from build123d import *

# Parameters (mm, degrees)
AUFSATZ_LINEAR_AUSTRAGEN1_DEPTH      = 10
SKIZZE6_R                            = 1.9
SKIZZE6_R_2                          = 11.25
SCHNITT_LINEAR_AUSTRAGEN4_DEPTH      = 67.632124385
SKIZZE7_W                            = 20.880821379
SKIZZE7_H                            = 5
SCHNITT_LINEAR_AUSTRAGEN5_DEPTH      = 87.970339772
VERRUNDUNG3_R                        = 15
SCHNITT_LINEAR_AUSTRAGEN6_DEPTH      = 69.731361244
SCHNITT_LINEAR_AUSTRAGEN6_DEPTH_BACK = 69.731361244
SKIZZE8_W                            = 10
SKIZZE8_H                            = 5
SKIZZE9_R                            = 1.7
SCHNITT_LINEAR_AUSTRAGEN7_DEPTH      = 10
AUFSATZ_LINEAR_AUSTRAGEN2_DEPTH      = 5


with BuildPart() as part:
    # Skizze1 → Aufsatz-Linear austragen1 (new body)
    with BuildSketch(Plane(origin=(0, 0, 0), x_dir=(1, 0, 0), z_dir=(0, 1, 0))):
        Polygon((-60, -4.8), (-22, -4.8), (-22, -16.8), (22, -16.8), (22, -4.8), (60, -4.8), (60, 15.2), (22, 15.2), (22, 27.2), (0, 27.2), (-22, 27.2), (-22, 15.2), (-60, 15.2), align=None)
    extrude(amount=AUFSATZ_LINEAR_AUSTRAGEN1_DEPTH)

    # Skizze6 → Schnitt-Linear austragen4 (cut, through all)
    with BuildSketch(Plane(origin=(0, 10, 0), x_dir=(1, 0, 0), z_dir=(0, 1, 0))):
        with Locations(Location((15.5, 20.7, 0), (0, 0, 270))):
            Circle(SKIZZE6_R)
        with Locations(Location((15.5, -10.3, 0), (0, 0, 270))):
            Circle(SKIZZE6_R)
        with Locations(Location((-15.5, -10.3, 0), (0, 0, 270))):
            Circle(SKIZZE6_R)
        with Locations(Location((-15.5, 20.7, 0), (0, 0, 270))):
            Circle(SKIZZE6_R)
        with Locations(Location((0, 5.2, 0), (0, 0, 270))):
            Circle(SKIZZE6_R_2)
    extrude(amount=-SCHNITT_LINEAR_AUSTRAGEN4_DEPTH, mode=Mode.SUBTRACT)

    # Skizze7 → Schnitt-Linear austragen5 (cut, through all)
    with BuildSketch(Plane.ZY.offset(22)):
        with Locations((-25.64041069, 2.5)):
            Rectangle(SKIZZE7_W, SKIZZE7_H)
    extrude(amount=-SCHNITT_LINEAR_AUSTRAGEN5_DEPTH, mode=Mode.SUBTRACT)

    # Verrundung3
    # the kernel refuses this fillet: 15 mm, written as the material it adds along each edge
    with BuildSketch(Plane(origin=(-22, 5, -15.2), x_dir=(0, 0, -1), z_dir=(0, 1, 0))) as verrundung3_piece_1:
        with BuildLine():
            CenterArc((15, 14.696938457), VERRUNDUNG3_R, 180, 78.463040967)
            Line((0, 14.696938457), (-0.3, 14.696938457))
            Line((-0.3, 14.696938457), (-0.3, 0))
            Line((-0.3, 0), (0, -0.3))
            ThreePointArc((0, -0.3), (6, -0.3), (11.94, -0.293938769))
            Line((11.94, -0.293938769), (12, 0))
        make_face()
    extrude(amount=5)
    with BuildSketch(Plane(origin=(-22, 0, 4.8), x_dir=(-1, 0, 0), z_dir=(0, 1, 0))) as verrundung3_piece_2:
        with BuildLine():
            CenterArc((14.696938457, 15), VERRUNDUNG3_R, 191.536959033, 78.463040967)
            Line((0, 12), (-0.293938769, 11.94))
            ThreePointArc((-0.293938769, 11.94), (-0.3, 6), (-0.3, 0))
            Line((-0.3, 0), (0, -0.3))
            Line((0, -0.3), (14.696938457, -0.3))
            Line((14.696938457, -0.3), (14.696938457, 0))
        make_face()
    extrude(amount=10)
    with BuildSketch(Plane(origin=(22, 0, 4.8), x_dir=(1, 0, 0), z_dir=(0, 1, 0))) as verrundung3_piece_3:
        with BuildLine():
            CenterArc((14.696938457, -15), VERRUNDUNG3_R, 90, 78.463040967)
            Line((0, -12), (-0.293938769, -11.94))
            ThreePointArc((-0.293938769, -11.94), (-0.3, -6), (-0.3, 0))
            Line((-0.3, 0), (0, 0.3))
            Line((0, 0.3), (14.696938457, 0.3))
            Line((14.696938457, 0.3), (14.696938457, 0))
        make_face()
    extrude(amount=10)
    with BuildSketch(Plane(origin=(22, 5, -15.2), x_dir=(1, 0, 0), z_dir=(0, 1, 0))) as verrundung3_piece_4:
        with BuildLine():
            CenterArc((14.696938457, 15), VERRUNDUNG3_R, 191.536959033, 78.463040967)
            Line((0, 12), (-0.293938769, 11.94))
            ThreePointArc((-0.293938769, 11.94), (-0.3, 6), (-0.3, 0))
            Line((-0.3, 0), (0, -0.3))
            Line((0, -0.3), (14.696938457, -0.3))
            Line((14.696938457, -0.3), (14.696938457, 0))
        make_face()
    extrude(amount=5)

    # Verrundung4
    # a fillet whose section is not a circle: 17 mm, written as the material it takes off along each edge
    with BuildSketch(Plane(origin=(-5.153882032, -55.537810403, -15.2), x_dir=(-0.4098221227148323, 0, 0.912165460721633), z_dir=(0, 1, 0))) as verrundung4_piece_1:
        with BuildLine():
            Bezier((14.018959465, 0), (3.694910003, -8.223980839), (9.10424934, -20.263868965), weights=[1, 0.223796354, 1])
            Line((9.10424934, -20.263868965), (0, 0))
            ThreePointArc((0, 0), (7.009479733, -2.450585595), (14.018959465, 0))
        make_face()
    extrude(amount=60.537810403, mode=Mode.SUBTRACT)
    with BuildSketch(Plane(origin=(5.153882032, -55.537810403, -15.2), x_dir=(0.40982212271483137, 0, 0.9121654607216333), z_dir=(0, 1, 0))) as verrundung4_piece_2:
        with BuildLine():
            Bezier((14.018959465, 0), (3.694910003, 8.223980839), (9.10424934, 20.263868965), weights=[1, 0.223796354, 1])
            Line((9.10424934, 20.263868965), (0, 0))
            ThreePointArc((0, 0), (7.009479733, 2.450585595), (14.018959465, 0))
        make_face()
    extrude(amount=60.537810403, mode=Mode.SUBTRACT)

    # Skizze8 → Schnitt-Linear austragen6 (cut, two sides: drawn at the far end of the back side and taken through both)
    with BuildSketch(Plane(origin=(0, 0, -15.2), x_dir=(-1, 0, 0), z_dir=(0, 0, -1)).offset(-SCHNITT_LINEAR_AUSTRAGEN6_DEPTH_BACK)):
        with Locations((-55, 2.5)):
            Rectangle(SKIZZE8_W, SKIZZE8_H)
        with Locations((55, 2.5)):
            Rectangle(SKIZZE8_W, SKIZZE8_H)
    extrude(amount=SCHNITT_LINEAR_AUSTRAGEN6_DEPTH + SCHNITT_LINEAR_AUSTRAGEN6_DEPTH_BACK, mode=Mode.SUBTRACT)

    # Skizze9 → Schnitt-Linear austragen7 (cut)
    with BuildSketch(Plane.XZ.offset(-5)):
        with Locations(Location((-55, -0.2, 0), (0, 0, 270))):
            Circle(SKIZZE9_R)
        with Locations(Location((-55, -10.2, 0), (0, 0, 90))):
            Circle(SKIZZE9_R)
        with Locations(Location((55, -10.2, 0), (0, 0, 270))):
            Circle(SKIZZE9_R)
        with Locations(Location((55, -0.2, 0), (0, 0, 90))):
            Circle(SKIZZE9_R)
    extrude(amount=-SCHNITT_LINEAR_AUSTRAGEN7_DEPTH, mode=Mode.SUBTRACT)

    # Skizze10 → Aufsatz-Linear austragen2 (add)
    with BuildSketch(Plane(origin=(0, 10, 0), x_dir=(1, 0, 0), z_dir=(0, 1, 0))):
        Polygon((-22, 27.2), (-20.360366379, 30.307150274), (-18.720732758, 27.2), align=None)
    extrude(amount=-AUFSATZ_LINEAR_AUSTRAGEN2_DEPTH)


solid = part.part
Verification items for the finished model (mm, model axes). A direction names the side the tool comes from. Give positions to 0.01 mm unless a question says otherwise; leave off trailing zeros. Write each loop counter-clockwise with the first axis right and the second up, starting at its lowest first coordinate (ties: lowest second). Pieces come first, ordered by that corner, then holes.
(1) Cross-section at D-D (z = -0.2). Enter the section's corners in (x, y), plus the area to 3 significant figures.
(2) Cross-section at B-B (z = 10.3). Enter the section's corners in (x, y).
(3) Gauge pin test, flat ends, axial feed: pin 1 (5.5 mm diameter, centred on x = 5, y = 6.5, fed in from -Z); pin 2 (5 mm diameter, centred on x = 37, y = 7, fed in from -Z); pin 3 (5.5 mm diameter, centred on x = 55, z = -0.2, fed in from -Y). Record the tip position at first contact, or that the pin passes through.
(4) Cross-section at A-A (y = 7). State how many separate pieces and enclosed holes the cut face has, plus the area to 3 significant figures.
(5) Material ranges on line 1 (X direction, y = 6, z = -0.2); line 2 (X direction, y = 8.25, z = -20.5); line 3 (Y direction, x = -53, z = -7), recorded low to high.
(6) Cross-section at C-C (x = -55). Enter the section's corners in (y, z), plus the area to 3 significant figures.
(7) Mould release check, pull along Z, two halves, no side actions. Record for faces 5 (the face through (-56.15, 7.46, -11.45)), 6 (the face through (55.07, 7.46, -8.5)), 7 (the face through (0, 5, 16.8)), 8 (the face through (1, 0, 8)): +Z half, -Z half, draft (parallel to the pull), parting line (faces both ways), or undercut.
(8) Access from +Z, -Z, +X, -X, +Y, -Y to the whole of each face (thin tool, end or side, straight path). Record for faces 1 (the face through (0, 5, -18)), 2 (the face through (43, 5, -15.2)), 3 (the face through (-46, 6, 4.8)), 4 (the face through (46, 6, 4.8)).
Worked out:
1. outline: (-60, 5) - (-56.7, 5) - (-56.7, 10) - (-60, 10) - close; (-53.3, 5) - (-50, 5) - (-50, 0) - (-10.08, 0) - (-10.08, 10) - (-53.3, 10) - close; (10.08, 0) - (50, 0) - (50, 5) - (53.3, 5) - (53.3, 10) - (10.08, 10) - close; (56.7, 5) - (60, 5) - (60, 10) - (56.7, 10) - close
1. area: 864 mm2
2. outline: (-25.09, 0) - (-17.4, 0) - (-17.4, 10) - (-25.09, 10) - close; (-13.6, 0) - (13.6, 0) - (13.6, 10) - (-13.6, 10) - close; (17.4, 0) - (25.09, 0) - (25.09, 10) - (17.4, 10) - close
3. pin 1: stops at z = -27.2
3. pin 2: stops at z = -15.36
3. pin 3: stops at y = 5
4. separate pieces: 1
4. enclosed holes: 9
4. area: 3,160 mm2
5. line 1: x = -60 to -56.7, -53.3 to -10.08, 10.08 to 53.3, 56.7 to 60
5. line 2: x = -25.26 to -17.39, -13.61 to 13.61, 17.39 to 25.26
5. line 3: y = 5 to 10
6. outline: (5, -15.2) - (10, -15.2) - (10, -11.9) - (5, -11.9) - close; (5, -8.5) - (10, -8.5) - (10, -1.9) - (5, -1.9) - close; (5, 1.5) - (10, 1.5) - (10, 4.8) - (5, 4.8) - close
6. area: 66.0 mm2
7. face 5: undercut
7. face 6: undercut
7. face 7: +Z half
7. face 8: draft
8. face 1: -Z, -Y
8. face 2: -Z, +X, -Y
8. face 3: +Z, -X, +Y, -Y
8. face 4: +Z, +X, +Y, -Y
